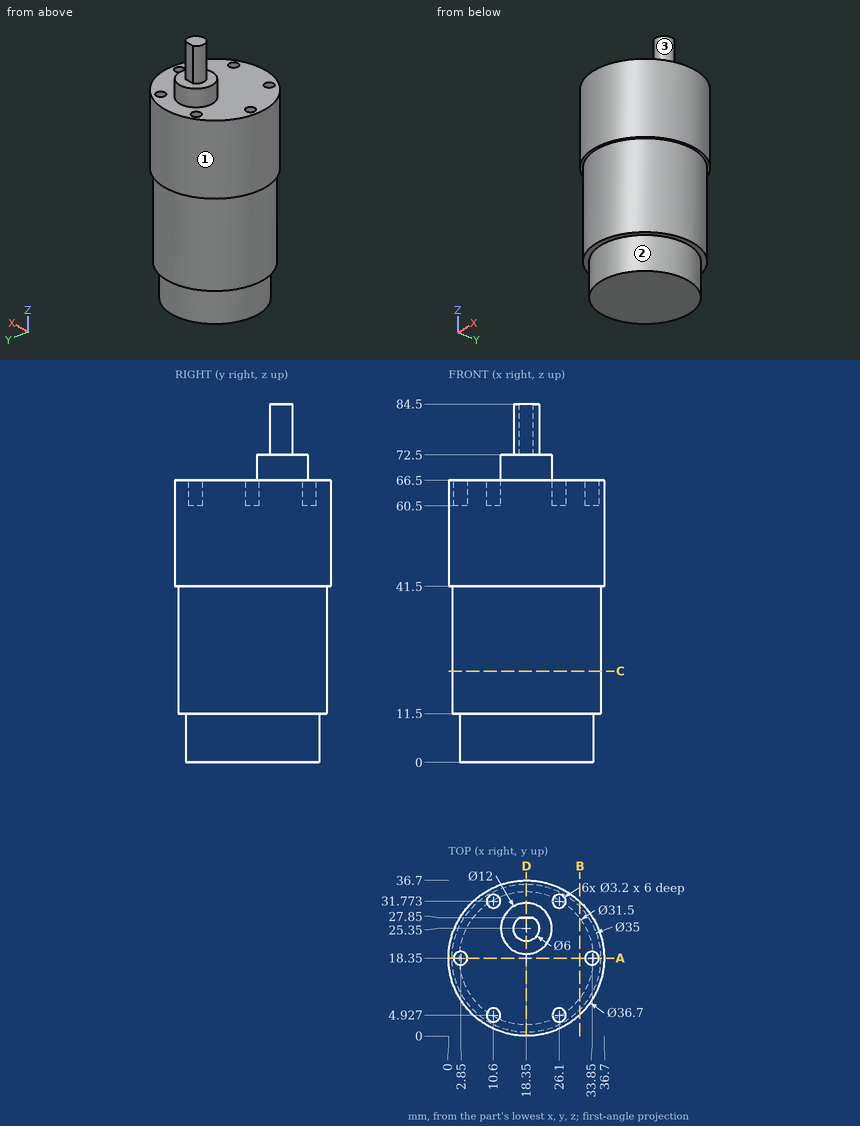
Design review of the part shown in the three views and the two pictorial views. Dimensions are in mm from the part's minimum x, y and z. A direction names the side the tool comes from. Give positions to 0.01 mm unless a question says otherwise; leave off trailing zeros. Write each loop counter-clockwise with the first axis right and the second up, starting at its lowest first coordinate (ties: lowest second). Pieces come first, ordered by that corner, then holes. Notation, with made-up numbers: M 27.25,4.25 L 83.25,4.25 A31 ccw 83.25,36.25 Z; hole C 27.5,13 d8. An arc over 180 degrees is marked long. Return JSON: item names as keys, results as strings. Group by question number.
Item 1: Clearance check with flat-ended pins moving along their axes: pin 1 Ø3 at (x, y) = (26.1, 4.93) entering from +Z; pin 2 Ø12 at (y, z) = (28, 35.5) entering from +X (1 decimal); pin 3 Ø8 at (y, z) = (7, 19.5) entering from -X. State where each tip first meets the part, or that it passes through.
Item 2: Wall thickness on line 1 along X through (y, z) = (18, 63); line 2 along Z through (x, y) = (27, 14.5); line 3 along Y through (x, z) = (26.1, 64.1): over which ranges is each line inside the solid? List them lowest first.
Item 3: Take a section at C-C (z = 21.5). Give the boundary of the cut face in (x, y), plus the area to 3 significant figures.
Item 4: Tool access review of the marked faces 1, 2 and 3: name each direction out of +Z, -Z, +X, -X, +Y, -Y from which nothing blocks a thin tool from reaching the whole face with its end or side.
Item 5: Take a section at B-B (x = 31). Give the boundary of the cut face in (y, z).
Item 6: Take a section at A-A (y = 18.35). Give the boundary of the cut face in (x, z), plus the area to 3 significant figures.
Item 7: Take a section at D-D (x = 18.35). Give the boundary of the cut face in (y, z).
Return value:
{
 "1": {"pin 1": "stops at z = 60.5", "pin 2": "stops at x = 35.5", "pin 3": "stops at x = 2.47"},
 "2": {"line 1": "x = 0 to 1.29, 4.41 to 32.29, 35.41 to 36.7", "line 2": "z = 0 to 66.5", "line 3": "y = 1.72 to 3.33, 6.53 to 30.17, 33.37 to 34.98"},
 "3": {"outline": "C 18.35,18.35 d35", "area": "962 mm2"},
 "4": {"face 1": "+Z, -Z", "face 2": "-Z", "face 3": "+Z"},
 "5": {"outline": "M 5.06,41.5 L 6.26,41.5 L 6.26,11.5 L 8.97,11.5 L 8.97,0 L 27.73,0 L 27.73,11.5 L 30.44,11.5 L 30.44,41.5 L 31.64,41.5 L 31.64,66.5 L 5.06,66.5 Z"},
 "6": {"outline": "M 0,41.5 L 0.85,41.5 L 0.85,11.5 L 2.6,11.5 L 2.6,0 L 34.1,0 L 34.1,11.5 L 35.85,11.5 L 35.85,41.5 L 36.7,41.5 L 36.7,66.5 L 35.45,66.5 L 35.45,60.5 L 32.25,60.5 L 32.25,66.5 L 4.45,66.5 L 4.45,60.5 L 1.25,60.5 L 1.25,66.5 L 0,66.5 Z", "area": "2,290 mm2"},
 "7": {"outline": "M 0,41.5 L 0.85,41.5 L 0.85,11.5 L 2.6,11.5 L 2.6,0 L 34.1,0 L 34.1,11.5 L 35.85,11.5 L 35.85,41.5 L 36.7,41.5 L 36.7,66.5 L 31.35,66.5 L 31.35,72.5 L 27.85,72.5 L 27.85,84.5 L 22.35,84.5 L 22.35,72.5 L 19.35,72.5 L 19.35,66.5 L 0,66.5 Z"}
}
